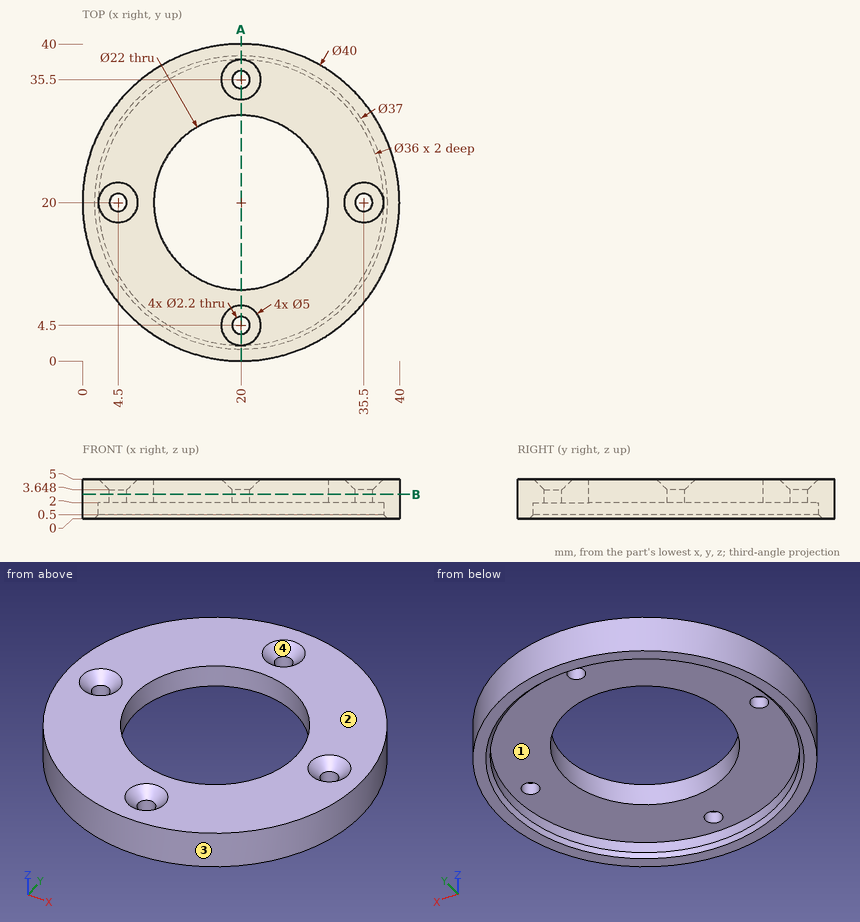
Check sheet for the drawn part. Datum: minimum x, y, z corner. Units: mm. Coordinates: 2 decimals unless noted, no trailing zeros. Write each loop counter-clockwise with the first axis right and the second up, starting at its lowest first coordinate (ties: lowest second). Pieces come first, ordered by that corner, then holes. Notation, with made-up numbers: (84.25, -30) - (112.25, -30) arc R15 cw to (112.25, -6) - close; hole circle Ø8 at (-1.5, 25.25). An arc over 180 degrees is marked (long way). Answer as a JSON object with one key per item and string values.
(1) Cross-section at B-B on z = 3.05. Record the cut outline in (x, y).
Report:
{"outline": "circle Ø40 at (20, 20); hole circle Ø2.2 at (4.5, 20); hole circle Ø22 at (20, 20); hole circle Ø2.2 at (20, 4.5); hole circle Ø2.2 at (20, 35.5); hole circle Ø2.2 at (35.5, 20)"}
(2) Gauge pin test, flat ends, axial feed: pin 1 Ø11 at (x, y) = (23.5, 16.5) entering from -Z; pin 2 Ø1 at (x, y) = (32.5, 30) entering from -Z; pin 3 Ø2 at (y, z) = (16.5, 2.5) entering from -X; pin 4 Ø3.5 at (x, y) = (4.5, 20) entering from +Z. Record the tip position at first contact, or that the pin passes through.
Report:
{"pin 1": "through", "pin 2": "z = 2", "pin 3": "x = 0.16", "pin 4": "z = 4.28"}
(3) Thickness scan on line 1 along Z through (x, y) = (13, 4); line 2 along X through (y, z) = (21, 2.4) (1 decimal); line 3 along Y through (x, z) = (20, 1.4). Record the ranges inside material, lowest first.
Report:
{"line 1": "2 to 5", "line 2": "0 to 4, 5 to 9, 31 to 35, 36 to 40", "line 3": "0 to 2, 38 to 40"}
(4) Cross-section at A-A on x = 20. Record the cut outline in (y, z).
Report:
{"outline": "(0, 0) - (1.5, 0) - (2, 0.5) - (2, 2) - (3.4, 2) - (3.4, 3.65) - (2, 5) - (0, 5) - close; (5.6, 2) - (9, 2) - (9, 5) - (7, 5) - (5.6, 3.65) - close; (31, 2) - (34.4, 2) - (34.4, 3.65) - (33, 5) - (31, 5) - close; (36.6, 2) - (38, 2) - (38, 0.5) - (38.5, 0) - (40, 0) - (40, 5) - (38, 5) - (36.6, 3.65) - close"}
(5) Mould release check, pull along Y, two halves, no side actions. Record for the marked faces 1, 2, 3 and 4: pulls with the +Y half, pulls with the -Y half, needs draft (parallel to the pull), parting line crosses it, or undercut.
Report:
{"face 1": "undercut", "face 2": "needs draft", "face 3": "parting line crosses it", "face 4": "undercut"}
